For this review, take the finished solid that the model builds, in its own axes (mm). Round coordinates to 2 decimals unless told otherwise and drop trailing zeros. Loops run counter-clockwise (first coordinate to the right, second up) from the corner with the lowest first, then second, coordinate; pieces in that order, holes last. Notation, with made-up numbers: M 26.5,22.5 L 47.5,22.5 A26 cw 47.5,58.5 Z; hole C 23,80.5 d2. An arc over 180 degrees is marked long. One line per question, with ' | ' between items. Start each with the question number.
1) For pin 1 Ø2 at (y, z) = (2.5, 2) entering from -X, flat-tipped, find the tip position at first contact; note if it passes through.
2) We need section A-A (x = 181). Give the boundary of the cut face in (y, z).
3) For probe 1 along Z at (x, y) = (-346, 0.95); probe 2 along X at (y, z) = (0.7, -6.5); probe 3 along Z at (x, y) = (102, 1.3), list the stretches that pass through material, from the lowest coordinate up. Write a range as from..to.
4) We need section B-B (y = 2.75). State how many separate pieces and enclosed holes the cut face has, and give its area (3 significant figures).
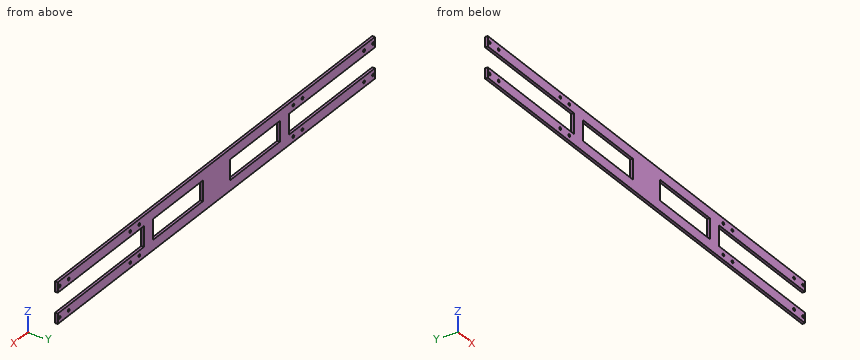
```python
from build123d import *

# Parameters (mm, degrees)
SKETCH_1_W                                 = 700
SKETCH_1_H                                 = 60
SKETCH_1_W_2                               = 280
SKETCH_1_H_2                               = 30
EXTRUDE_1_DEPTH                            = 4
SKETCH_2_W                                 = 190
SKETCH_2_H                                 = 30
CUT_EXTRUDE_1_DEPTH                        = 4
SKETCH_3_R                                 = 2
CUT_EXTRUDE_2_DEPTH                        = 4
MIRROR_2_AT_THE_SECOND_PLANE_COPY_1_SKET_R = 2
MIRROR_2_AT_THE_SECOND_PLANE_COPY_1_DEPTH  = 4
SKETCH_4_W                                 = 60
SKETCH_4_H                                 = 30
EXTRUDE_2_DEPTH                            = 4


with BuildPart() as part:
    # 草图1 → 凸台-拉伸1 (new body)
    with BuildSketch(Plane(origin=(0, 0, 0), x_dir=(1, 0, 0), z_dir=(0, 1, 0))):
        Rectangle(SKETCH_1_W, SKETCH_1_H)
        Rectangle(SKETCH_1_W_2, SKETCH_1_H_2, mode=Mode.SUBTRACT)
    extrude(amount=EXTRUDE_1_DEPTH)

    # 草图2 → 切除-拉伸1 (cut)
    with BuildSketch(Plane(origin=(0, 4, 0), x_dir=(1, 0, 0), z_dir=(0, 1, 0))):
        with Locations((-255, 0)):
            Rectangle(SKETCH_2_W, SKETCH_2_H)
    cut_extrude_1 = extrude(amount=-CUT_EXTRUDE_1_DEPTH, mode=Mode.SUBTRACT)

    # 镜向1: 切除-拉伸1 across plane
    add(cut_extrude_1.mirror(Plane(origin=(0, 0, 0), x_dir=(0, 0, 1), z_dir=(1, 0, 0))), mode=Mode.SUBTRACT)

    # 草图3 → 切除-拉伸2 (cut)
    with BuildSketch(Plane(origin=(0, 4, 0), x_dir=(1, 0, 0), z_dir=(0, 1, 0))):
        with Locations(Location((-190, 22.5, 0), (0, 0, 270))):
            Circle(SKETCH_3_R)
        with Locations(Location((-170, 22.5, 0), (0, 0, 270))):
            Circle(SKETCH_3_R)
        with Locations(Location((-346, 22.5, 0), (0, 0, 270))):
            Circle(SKETCH_3_R)
        with Locations(Location((-326, 22.5, 0), (0, 0, 270))):
            Circle(SKETCH_3_R)
    cut_extrude_2 = extrude(amount=-CUT_EXTRUDE_2_DEPTH, mode=Mode.SUBTRACT)

    # 镜向2: 切除-拉伸2 across plane
    add(cut_extrude_2.mirror(Plane(origin=(0, 0, 0), x_dir=(0, 0, 1), z_dir=(1, 0, 0))), mode=Mode.SUBTRACT)

    # 镜向2 at the second plane: 切除-拉伸2 across plane
    add(cut_extrude_2.mirror(Plane.XY), mode=Mode.SUBTRACT)

    # 镜向2 at the second plane copy 1 sket → 镜向2 at the second plane copy 1 (cut)
    with BuildSketch(Plane(origin=(0, 4, 0), x_dir=(-1, 0, 0), z_dir=(0, 1, 0))):
        with Locations(Location((-190, 22.5, 0), (0, 0, 270))):
            Circle(MIRROR_2_AT_THE_SECOND_PLANE_COPY_1_SKET_R)
        with Locations(Location((-170, 22.5, 0), (0, 0, 270))):
            Circle(MIRROR_2_AT_THE_SECOND_PLANE_COPY_1_SKET_R)
        with Locations(Location((-346, 22.5, 0), (0, 0, 270))):
            Circle(MIRROR_2_AT_THE_SECOND_PLANE_COPY_1_SKET_R)
        with Locations(Location((-326, 22.5, 0), (0, 0, 270))):
            Circle(MIRROR_2_AT_THE_SECOND_PLANE_COPY_1_SKET_R)
    extrude(amount=-MIRROR_2_AT_THE_SECOND_PLANE_COPY_1_DEPTH, mode=Mode.SUBTRACT)

    # 草图4 → 凸台-拉伸2 (add)
    with BuildSketch(Plane(origin=(0, 4, 0), x_dir=(1, 0, 0), z_dir=(0, 1, 0))):
        Rectangle(SKETCH_4_W, SKETCH_4_H)
    extrude(amount=-EXTRUDE_2_DEPTH)


solid = part.part
```
Answers below:
1) pin 1: x = -160
2) outline: M 0,-30 L 4,-30 L 4,-15 L 0,-15 Z; M 0,15 L 4,15 L 4,30 L 0,30 Z
3) probe 1: -30..-24.5, -20.5..-15, 15..20.5, 24.5..30 | probe 2: -160..-140, -30..30, 140..160 | probe 3: -30..-15, 15..30
4) separate pieces: 1 | enclosed holes: 18 | area: 23,800 mm^2
